Autodesk Inventor part; units mm, degrees
ref_plane "Work Plane1" through (29, 0, 0) normal (0, -1, 0) x (1, 0, 0)
ref_plane "YZ Plane" through (0, 0, 0) normal (1, 0, 0) x (0, 1, 0)
ref_plane "XZ Plane" through (0, 0, 0) normal (0, 1, 0) x (-1, 0, 0)
sketch "Sketch1" plane through (0, 0, 0) normal (0, 0, 1) x (1, 0, 0)
  line L0 (0.2709, 0) -> (12.7, 0)
  line L1 (12.7, 0) -> (12.7, 2.413)
  line L2 (12.7, 2.413) -> (2.1084, 2.413)
  line L3 (2.1084, 2.413) -> (0.0001, 2.413)
  line L4 (0.0001, 2.413) -> (0, 2.413)
  line L5 (0, 2.413) -> (0, 4.5847)
  line L6 (0, 4.5847) -> (-2.5654, 4.5847)
  line L7 (-2.5654, 4.5847) -> (-2.5654, 1.8331)
  line L8 (-2.5654, 1.8331) -> (-0.7874, 1.8331)
  line L9 (-0.7874, 1.8331) -> (0.2709, 0)
  line L10 (-5.6185, 0) -> (15.7531, 0)
  line L11 (0, -0.9169) -> (0, 5.5016)
  line L12 (2.1084, 2.413) -> (0, 2.413) construction
  dimension "d1" = 10.5916
  dimension "d2" = 2.1083
  dimension "d3" = 2.5654
  dimension "d4" = 1.778
  dimension "d5" = 60
  dimension "d6" = 4.826
  dimension "d7" = 4.826
  dimension "d8" = 3.6662
  dimension "d9" = 9.1694
  dimension "d26" = 12.7
revolve "Body" add sketch "Sketch1" angle 360 about axis through (0.2709, 0, 0) along (1, 0, 0) contours L9 L11 L3 L2 L1 L0 | L9 L8 L7 L6 L5 L11
sketch "Sketch2" plane through (-2.5654, 0, 0) normal (-1, 0, 0) x (0, 0, 1)
  circle A0 centre (0, 0) radius 1.8331
  line L0 (0, -6.4186) -> (0, 6.4186)
  line L1 (-6.4186, 0) -> (6.4186, 0)
  line L2 (1.8331, 0) -> (0.9165, -1.5875)
  line L3 (0.9165, -1.5875) -> (-0.9165, -1.5875)
  line L4 (-0.9165, -1.5875) -> (-1.8331, 0)
  line L5 (-1.8331, 0) -> (-0.9165, 1.5875)
  line L6 (-0.9165, 1.5875) -> (0.9165, 1.5875)
  line L7 (0.9165, 1.5875) -> (1.8331, 0)
extrude "Slot" add sketch "Sketch2" against normal up to next contours L7 A0 | A0 L2 | L6 L0 A0 | A0 L0 L3 | L0 L6 A0 | A0 L3 L0 | L4 A0 | A0 L5
fillet "Fillet1" radius 2.3114 1 edges at (-2.5654, -4.5847, 0)
thread "Thread"
chamfer "Chamfer1" distance 0.6492 distance2 0.6492 1 edges at (12.7, -2.413, 0) measured on face at (12.7, -0.2686, 0.7084)
ref_plane "Work Plane1" through (29, 0, 0) normal (0, -1, 0) x (1, 0, 0)
fillet "Fillet2" radius 0.1 1 edges at (0.0001, -2.413, 0)
equation "\"d1\" = GEL"
equation "\"d3\" = KOH"
equation "\"d4\" = INTI"
equation "\"d6\" = GD"
equation "\"d7\" = BDM"
equation "\"d8\" = 1.1547 * SW"
equation "\"d9\" = KOD"
equation "\"d26\" = NLG"
equation "\"d30\" = R"
equation "\"d17\" = RR"
equation "\"d13\" = GEL"
equation "\"d15\" = -0.5 * SPD + 0.5 * GD"
equation "\"d16\" = GUL"
equation "\"GD\" = NND"
equation "\"NLG\" = 12.7"
equation "\"GEL\" = 10.5916"
equation "\"KOD\" = 9.1694"
equation "\"KOH\" = 2.5654"
equation "\"INTI\" = 1.778"
equation "\"GAL\" = 2.1082"
equation "\"GUL\" = 0.64922"
equation "\"BDM\" = NND"
equation "\"SW\" = 3.175"
equation "\"RR\" = 2.3114"
equation "\"SPD\" = 3.52755"
equation "\"R\" = 0.1"
equation "\"TOA\" = 30deg"
equation "\"GD1\" = SPD"
equation "\"THREADDIA\" = 4.826"
equation "\"KOH1\" = 0.508"
equation "\"NND\" = 4.826"
equation "\"E0\" = 3.66725"
properties part number "ANSI B18.3 - 10 - 24 x 1/2"
Read the model definition and answer for the solid it produces. Units are mm, in the model's axes. A direction names the side the tool comes from. Coordinates: 2 decimals unless noted, no trailing zeros. Loops run counter-clockwise (first coordinate to the right, second up) from the corner with the lowest first, then second, coordinate; pieces in that order, holes last. Notation, with made-up numbers: (29, 7.5) - (34, 7.5) arc R29 cw to (34, 30.5) - close; hole circle Ø6 at (85.25, 62). An arc over 180 degrees is marked (long way). Answer in a Markdown table with one row per item.
Q1. Find section A-A on x = 1.5. Write down the section's boundary in (y, z).
Here are the results:
| item | result |
|---|---|
| outline | circle Ø4.83 at (0, 0) |
Q2. The mould has two halves that part along Z. Classify faces 4 (the cylindrical face through (5.992, -1.915, 1.468)), 5 (the flat face through (-1.62, -0.8, -1.37)), 6 (the flat face through (-2.565, -2, 0)): pulls with the +Z half, pulls with the -Z half, needs draft (parallel to the pull), parting line crosses it, or undercut.
Here are the results:
| item | result |
|---|---|
| face 4 | parting line crosses it |
| face 5 | undercut |
| face 6 | needs draft |
Q3. Given P1, Ø3, axis at x = 7.5, y = 0, coming from the -Z side; P2, Ø1.5, axis at x = 4.5, y = -0.5, coming from the +Z side; P3, Ø2, axis at x = -2, z = 0.5, coming from the -Y side, each flat-ended and moving along its own axis, determine where each tip first touches the part or whether it passes through.
Here are the results:
| item | result |
|---|---|
| P1 | stops at z = -2.41 |
| P2 | stops at z = 2.41 |
| P3 | stops at y = -4.44 |
Q4. For faces 1 (the conical face through (0, -1, 3)), 2 (the flat face through (12.7, 0, 0)), 3 (the flat face through (-1.619, 0.783, -1.381)), determine the directions among +Z, -Z, +X, -X, +Y, -Y from which every point of the face is accessible in a straight line to the end or side of a thin tool.
Here are the results:
| item | result |
|---|---|
| face 1 | +X |
| face 2 | +Z, -Z, +X, +Y, -Y |
| face 3 | -X |
Q5. Straight lines are drawn through the part: line 1 along Z through (x, y) = (9.75, 0); line 2 along X through (y, z) = (0.75, -3); line 3 along X through (y, z) = (0.5, 1.5). For each, find the intervals that lie inside material, in ascending order. Write a range as [from, to].
Here are the results:
| item | result |
|---|---|
| line 1 | z = [-2.41, 2.41] |
| line 2 | x = [-2.42, 0] |
| line 3 | x = [-0.64, 12.7] |
